Here's the drawing with two shaded views (mm, measured from the low corner). I have some questions. A direction names the side the tool comes from. Round coordinates to 2 decimals unless told otherwise and drop trailing zeros. Loops run counter-clockwise (first coordinate to the right, second up) from the corner with the lowest first, then second, coordinate; pieces in that order, holes last.
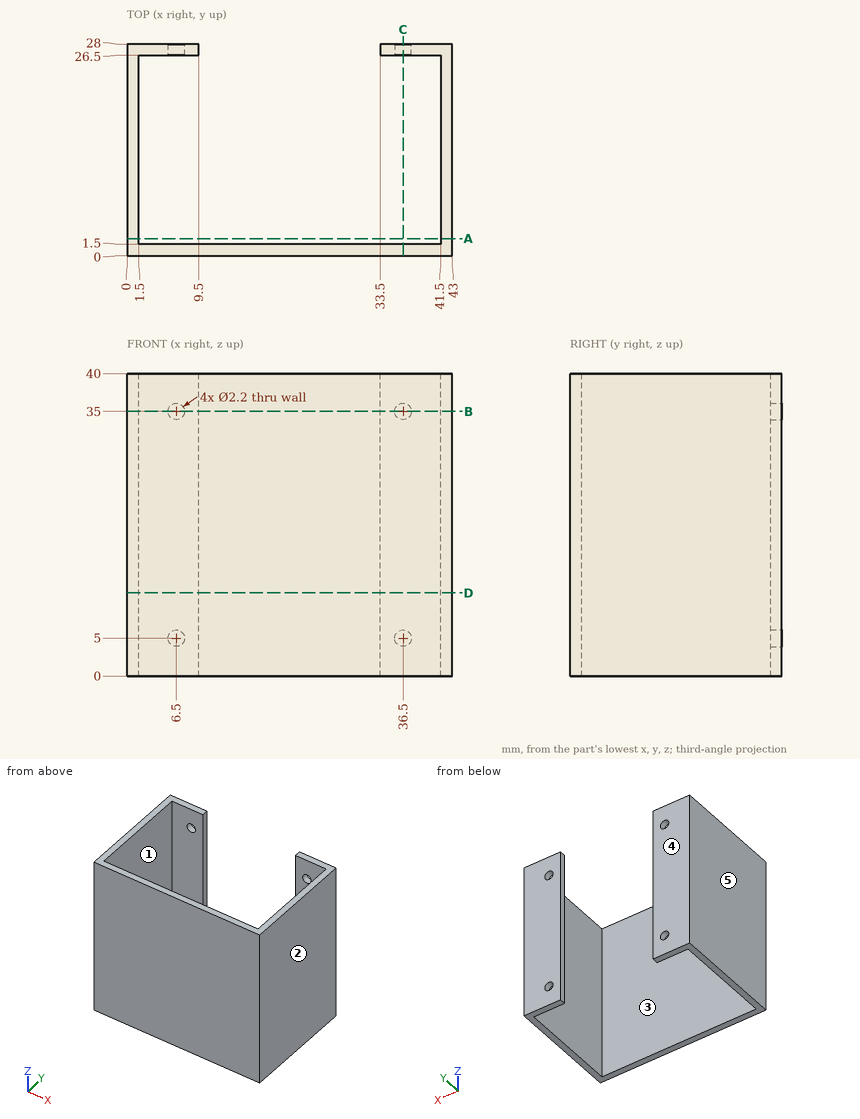
Item 1: Will this pin go through, and if not, where does the flat tip stop? pin 1 (8 mm diameter, centred on x = 12, y = 19, fed in from +Z).
Results list:
pin 1: passes through
Item 2: We'd pull the mould along X, two halves only. Please class the marked faces 3, 4 and 5: released by +X, released by -X, zero draft, split by the parting line, or undercut.
Results list:
face 3: undercut
face 4: zero draft
face 5: released by -X
Item 3: If we section it at D-D, the plane z = 11: Please give me the cut outline in (x, y).
Results list:
outline: (0, 0) - (43, 0) - (43, 28) - (33.5, 28) - (33.5, 26.5) - (41.5, 26.5) - (41.5, 1.5) - (1.5, 1.5) - (1.5, 26.5) - (9.5, 26.5) - (9.5, 28) - (0, 28) - close
Item 4: For the marked faces 1 and 2, which set-ups out of +Z, -Z, +X, -X, +Y, -Y let a thin tool reach every point of the face, with its end or its side?
Results list:
face 1: +Z, -Z
face 2: +Z, -Z, +X, +Y, -Y
Item 5: If we section it at C-C, the plane x = 36.5: Please give me the cut outline in (y, z).
Results list:
outline: (0, 0) - (1.5, 0) - (1.5, 40) - (0, 40) - close; (26.5, 0) - (28, 0) - (28, 3.9) - (26.5, 3.9) - close; (26.5, 6.1) - (28, 6.1) - (28, 33.9) - (26.5, 33.9) - close; (26.5, 36.1) - (28, 36.1) - (28, 40) - (26.5, 40) - close
Item 6: If we section it at A-A, the plane y = 2.25: Please give me the cut outline in (x, z), then the cut area to 3 significant figures.
Results list:
outline: (0, 0) - (1.5, 0) - (1.5, 40) - (0, 40) - close; (41.5, 0) - (43, 0) - (43, 40) - (41.5, 40) - close
area: 120 mm2
Item 7: If we section it at B-B, the plane z = 35: Please give me the cut outline in (x, y).
Results list:
outline: (0, 0) - (43, 0) - (43, 28) - (37.6, 28) - (37.6, 26.5) - (41.5, 26.5) - (41.5, 1.5) - (1.5, 1.5) - (1.5, 26.5) - (5.4, 26.5) - (5.4, 28) - (0, 28) - close; (7.6, 26.5) - (9.5, 26.5) - (9.5, 28) - (7.6, 28) - close; (33.5, 26.5) - (35.4, 26.5) - (35.4, 28) - (33.5, 28) - close
Item 8: If I drill on line 1 along Z through (x, y) = (36.5, 27.5); line 2 along X through (y, z) = (17.5, 35); line 3 along Y through (x, z) = (37.5, 18), over which ranges is the centre line in solid material (lowest first)?
Results list:
line 1: z = 0 to 3.9, 6.1 to 33.9, 36.1 to 40
line 2: x = 0 to 1.5, 41.5 to 43
line 3: y = 0 to 1.5, 26.5 to 28
